from build123d import *

# Parameters (mm, degrees)
F1_DEPTH = 1.778
F2_W     = 13.335
F2_H     = 8.89
F2_W_2   = 15.875
F2_H_2   = 12.7
F3_DEPTH = 9.525
F4_R     = 1.5875
F5_DEPTH = 1.778


with BuildPart() as f1:
    # F0 (on Front) → F1 (new body)
    with BuildSketch(Plane.XZ):
        Polygon((29.10832, 24.370352), (-35.40768, 24.370352), (-35.40768, -28.969648), (29.10832, -28.969648), (29.10832, -26.429648), (32.137258, -24.022085), (32.41032, 9.638352), (30.63232, 11.416352), (30.63232, 22.846352), align=None)
    extrude(amount=F1_DEPTH)

    # F2 (on Front) → F3 (join)
    with BuildSketch(Plane.XZ):
        with Locations((-30.537364, -21.481267)):
            Rectangle(F2_W, F2_H)
        with Locations((-31.807364, 9.633733)):
            Rectangle(F2_W_2, F2_H_2)
    extrude(amount=F3_DEPTH)

    # F4 (on Front) → F5 (cut)
    with BuildSketch(Plane.XZ):
        with Locations((-20.330156, 22.014147)):
            Circle(F4_R)
        with Locations((-21.484396, -26.541674)):
            Circle(F4_R)
        with Locations((30.017542, 6.413083)):
            Circle(F4_R)
        with Locations((30.00577, -21.418037)):
            Circle(F4_R)
    extrude(amount=F5_DEPTH, mode=Mode.SUBTRACT)


solid = f1.part
The model under review builds one solid part; all positions refer to its coordinate system, in mm. A direction names the side the tool comes from. Coordinates: 2 decimals unless noted, no trailing zeros. Loops run counter-clockwise (first coordinate to the right, second up) from the corner with the lowest first, then second, coordinate; pieces in that order, holes last. Notation, with made-up numbers: (80.25, -5) -> (133.25, -5) arc R30 ccw to (133.25, 23) -> close; hole circle Ø2 at (56.5, 13). An arc over 180 degrees is marked (long way). Use a Markdown table: item, result. Add a question column.
1. Draft analysis for pull direction Z (two halves, no side actions). For faces 1 (the face through (-23.87, -6, 10)), 2 (the face through (-3, -1, 24.37)), 3 (the face through (-31, -6, -17.036)), 4 (the face through (-4, -1, -28.97)), state which applies: pulls with the +Z half, pulls with the -Z half, needs draft (parallel to the pull), parting line crosses it, or undercut.
2. Machinability: for faces 5 (the face through (-37.205, -5, -22)), 6 (the face through (-23.87, -6, -22)), 7 (the face through (29.108, -1, -28)), which of the approach directions +Z, -Z, +X, -X, +Y, -Y give a long, thin tool a straight path to every point of the face, cutting with its end or side? Answer none if there is none.
3. Add section D-D on x = -9. Write out the cut boundary in (y, z).
4. To check wall thickness, follow line 1 (Z direction, x = -25.5, y = -8.75); line 2 (Y direction, x = 18, z = 4); line 3 (X direction, y = -1, z = 11.5). State the ranges of each line that lie inside material, in increasing order.
5. Add section A-A on y = -8.5. Write out the cut boundary in (x, z).
6. Clearance check with flat-ended pins moving along their axes: pin 1 Ø0.9 at (y, z) = (-1.5, -8) entering from -X; pin 2 Ø1.5 at (x, z) = (8.5, 17) entering from -Y; pin 3 Ø1.4 at (y, z) = (-0.5, -27.5) entering from +X. State where each tip first meets the part, or that it passes through.
7. Add section B-B on x = -27. Write out the cut boundary in (y, z) (3 decimals), plus the area to 3 significant figures.
8. Add section C-C on z = 17. Write out the cut boundary in (x, y), plus the area to 3 significant figures.
Returned:
| question | item | result |
|---|---|---|
| 1 | face 1 | needs draft |
| 1 | face 2 | pulls with the +Z half |
| 1 | face 3 | undercut |
| 1 | face 4 | pulls with the -Z half |
| 2 | face 5 | -Z, -X, +Y, -Y |
| 2 | face 6 | +Z, -Z, +X, -Y |
| 2 | face 7 | -Z, +X, +Y, -Y |
| 3 | outline | (-1.78, -28.97) -> (0, -28.97) -> (0, 24.37) -> (-1.78, 24.37) -> close |
| 4 | line 1 | z = -25.93 to -17.04, 3.28 to 15.98 |
| 4 | line 2 | y = -1.78 to 0 |
| 4 | line 3 | x = -39.74 to 30.63 |
| 5 | outline | (-39.74, 3.28) -> (-23.87, 3.28) -> (-23.87, 15.98) -> (-39.74, 15.98) -> close; (-37.2, -25.93) -> (-23.87, -25.93) -> (-23.87, -17.04) -> (-37.2, -17.04) -> close |
| 6 | pin 1 | stops at x = -35.41 |
| 6 | pin 2 | stops at y = -1.78 |
| 6 | pin 3 | stops at x = 29.11 |
| 7 | outline | (-9.525, -25.926) -> (-1.778, -25.926) -> (-1.778, -28.97) -> (0, -28.97) -> (0, 24.37) -> (-1.778, 24.37) -> (-1.778, 15.984) -> (-9.525, 15.984) -> (-9.525, 3.284) -> (-1.778, 3.284) -> (-1.778, -17.036) -> (-9.525, -17.036) -> close |
| 7 | area | 262 mm² |
| 8 | outline | (-35.41, -1.78) -> (30.63, -1.78) -> (30.63, 0) -> (-35.41, 0) -> close |
| 8 | area | 117 mm² |
